CAD build for the part. Positions are in the model's coordinates, mm. Face numbers are marked on the shaded views. Round coordinates to 2 decimals unless told otherwise and drop trailing zeros. Loops run counter-clockwise (first coordinate to the right, second up) from the corner with the lowest first, then second, coordinate; pieces in that order, holes last. Notation, with made-up numbers: (-24.5, -34.5) -> (-13.5, -34.5) arc R22 cw to (-13.5, -9.5) -> close; hole circle Ø5 at (45, -4). An arc over 180 degrees is marked (long way). Answer as CSV lines item,"result".
```python
from build123d import *

# Parameters (mm, degrees)
F0_R      = 11
F1_DEPTH  = 9.6
F2_R      = 10.2
F3_DEPTH  = 8.6
F4_R      = 1.4
F5_DEPTH  = 12.5
F8_R      = 1.4
F9_DEPTH  = 12.5
F12_DEPTH = 2.8
F13_R     = 3.5
F14_DEPTH = 1


with BuildPart() as f1:
    # F0 (on Top) → F1 (new body)
    with BuildSketch(Plane.XY):
        Circle(F0_R)
    extrude(amount=F1_DEPTH)

    # F2 (on face) → F3 (cut)
    with BuildSketch(Plane.XY.offset(9.6)):
        Circle(F2_R)
    extrude(amount=-F3_DEPTH, mode=Mode.SUBTRACT)

    # F4 (on Front) → F5 (cut, symmetric)
    with BuildSketch(Plane.XZ):
        with Locations((0, 3.3)):
            Circle(F4_R)
    extrude(amount=F5_DEPTH, both=True, mode=Mode.SUBTRACT)

    # F8 (on line) → F9 (cut, symmetric)
    with BuildSketch(Plane(origin=(0, 0, 0), x_dir=(-0.7071067812, 0.7071067812, 0), z_dir=(0.7071067812, 0.7071067812, 0))):
        with Locations((0, 3.3)):
            Circle(F8_R)
    extrude(amount=F9_DEPTH, both=True, mode=Mode.SUBTRACT)

    # F11 (on offset) → F12 (cut)
    with BuildSketch(Plane.XY.offset(1.9)):
        Polygon((0, 13.7625831805), (0, 0), (9.7316158935, 9.7316158935), align=None)
        Polygon((0, -13.7625831805), (0, 0), (-9.7316158935, -9.7316158935), align=None)
    extrude(amount=F12_DEPTH, mode=Mode.SUBTRACT)

    # F13 (on face) → F14 (cut, through all)
    with BuildSketch(Plane.XY.offset(1)):
        Circle(F13_R)
    extrude(amount=-F14_DEPTH, mode=Mode.SUBTRACT)


solid = f1.part
```
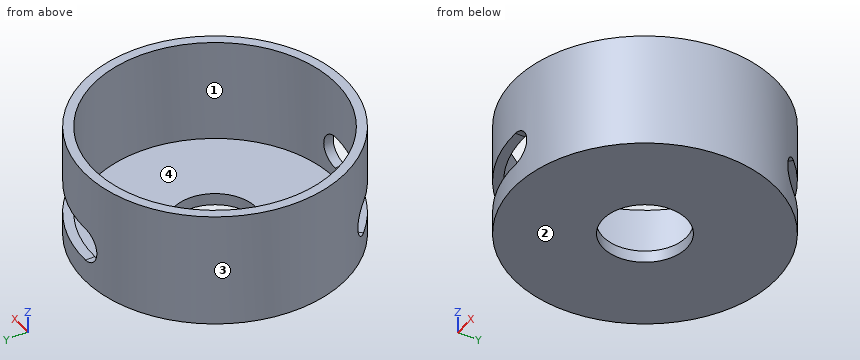
Q1. Slice it at B-B, the plane x = 4. Give the cut face in (y, z).
Results:
outline,"(-10.25, 0) -> (10.25, 0) -> (10.25, 1.9) -> (9.38, 1.9) -> (9.38, 1) -> (-9.38, 1) -> (-9.38, 9.6) -> (-10.25, 9.6) -> close; (9.38, 4.7) -> (10.25, 4.7) -> (10.25, 9.6) -> (9.38, 9.6) -> close"
Q2. Probe L1, parallel to Y at x = 0, z = 0.7; L2, parallel to Z at x = -6.25, y = 5.25; L3, parallel to X at y = 0.25, z = 4.5. List the from-to ranges inside material, lowest first. Write a range as [from, to].
Results:
L1,"[-11, -3.5], [3.5, 11]"
L2,"[0, 1]"
L3,"[-11, -10.2], [10.2, 11]"
Q3. Slice it at C-C, the plane z = 3.3. Give the cut face in (x, y), and give its area (3 significant figures).
Results:
outline,"(-8.7, -6.72) -> (-8.13, -6.15) arc R10.2 cw to (-1.4, 10.1) -> (-1.4, 10.91) arc R11 ccw to start; (1.4, -10.91) arc R11 ccw to (8.7, 6.72) -> (8.13, 6.15) arc R10.2 cw to (1.4, -10.1) -> close"
area,"35.5 mm2"
Q4. Drop flat-ended pins along their axis: pin 1 Ø6 at (x, y) = (4.5, 1.5) entering from +Z; pin 2 Ø2 at (y, z) = (-6.5, 5.5) entering from -X; pin 3 Ø2 at (y, z) = (-3.5, 5) entering from +X. Give the stop position or say it passes through.
Results:
pin 1,"z = 1"
pin 2,"x = -9.53"
pin 3,"x = 10.71"
Q5. Slice it at A-A, the plane y = 0. Give the cut face in (x, z).
Results:
outline,"(-11, 0) -> (-3.5, 0) -> (-3.5, 1) -> (-10.2, 1) -> (-10.2, 9.6) -> (-11, 9.6) -> close; (3.5, 0) -> (11, 0) -> (11, 9.6) -> (10.2, 9.6) -> (10.2, 1) -> (3.5, 1) -> close"
Q6. Slice it at D-D, the plane y = -5.25. Give the cut face in (x, z), and give its area (3 significant figures).
Results:
outline,"(-9.67, 0) -> (9.67, 0) -> (9.67, 9.6) -> (8.75, 9.6) -> (8.75, 1) -> (-8.75, 1) -> (-8.75, 9.6) -> (-9.67, 9.6) -> close"
area,"35.2 mm2"
Q7. Two-plate mould, pull along X, no slides. Class the marked faces 1, 2, 3 and 4: pulls with the +X half, pulls with the -X half, needs draft (parallel to the pull), parting line crosses it, or undercut.
Results:
face 1,"undercut"
face 2,"needs draft"
face 3,"parting line crosses it"
face 4,"undercut"
